Job drawing, mm, ordinate dimensions from the low corner. One solid piece. A direction names the side the tool comes from. Round coordinates to 2 decimals unless told otherwise and drop trailing zeros. Order: outer loops, then holes, each group sorted by start corner. A loop starts at its lowest first (then second) coordinate and runs counter-clockwise, first axis right, second up. Notation, with made-up numbers: (74, -30) -> (95, -30) arc R18 cw to (95, 2) -> close; hole circle Ø4 at (-23, 3.5). An arc over 180 degrees is marked (long way). Return JSON: item names as keys, results as strings. Group by question number.
Q1. Which spindle directions (+Z, -Z, +X, -X, +Y, -Y) get a long thin tool onto all of the face, cutting with end or side? Do the marked faces 4, 5 and 6. Say none if no direction does.
Q2. Mould opens along Y. For the marked faces 1, 2 and 3 say: +Y half, -Y half, draft (parallel to the pull), parting line (faces both ways), or undercut.
Q3. Flat gauge pins, fed straight in: pin 1 (7.5 mm diameter, centred on x = 60, y = 17.5, fed in from +Z); pin 2 (5 mm diameter, centred on y = 8, z = 6, fed in from +X); pin 3 (1.5 mm diameter, centred on y = 21, z = 9, fed in from -X). Where does each tip first touch, or does it go through?
Q4. Cut at B-B (z = 33.5). Write the cut outline in (x, y).
Q5. Cut at D-D (y = 23). Write the cut outline in (x, z), then the cut area to 3 significant figures.
Q6. Cut at A-A (y = 14). Write the cut outline in (x, z).
Q7. Probe line 1 along Z through (x, y) = (44.25, 12.7) (3 decimals); line 2 along X through (y, z) = (8.75, 8); line 3 along X through (y, z) = (19, 21.5). List the from-to ranges inside material, lowest first.
Q8. Cut at C-C (x = 14). Write the cut outline in (y, z), then the cut area to 3 significant figures.
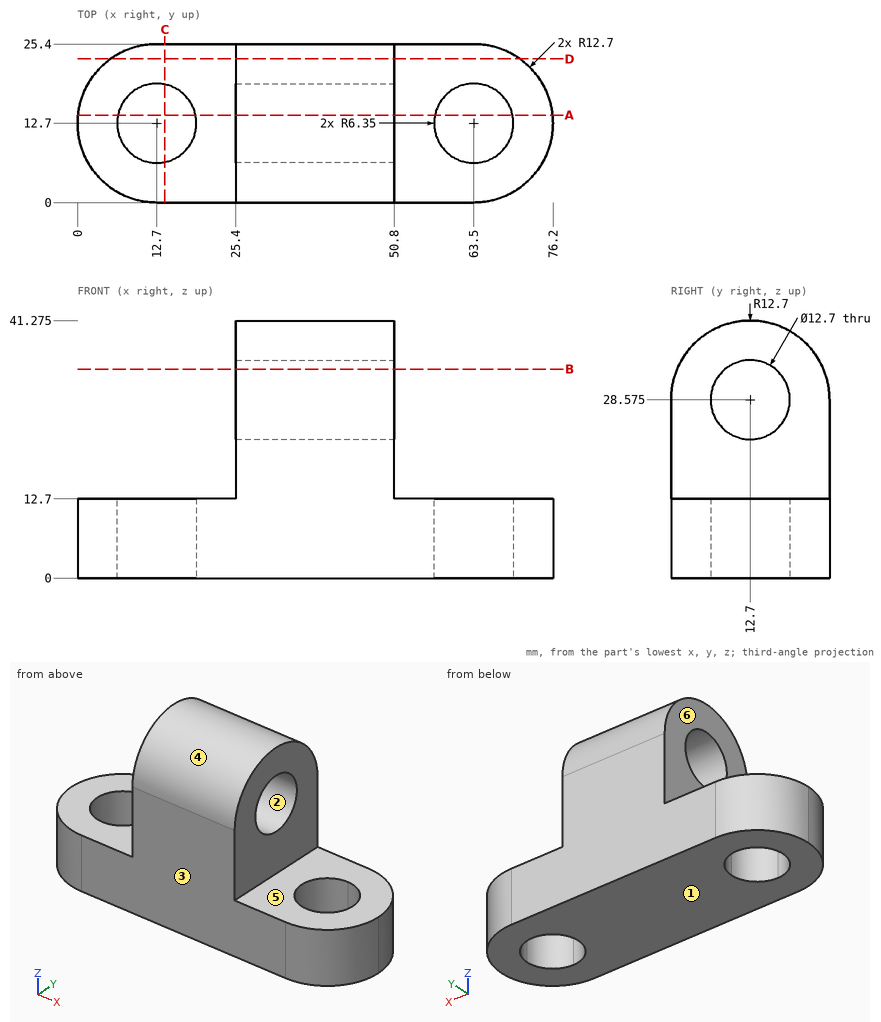
Solution:
{
 "1": {"face 4": "+Z, +X, -X", "face 5": "+Z, +X, +Y, -Y", "face 6": "+Z, -X, +Y, -Y"},
 "2": {"face 1": "draft", "face 2": "undercut", "face 3": "-Y half"},
 "3": {"pin 1": "stops at z = 12.7", "pin 2": "stops at x = 76.01", "pin 3": "stops at x = 2.49"},
 "4": {"outline": "(25.4, 0.99) -> (50.8, 0.99) -> (50.8, 8.69) -> (25.4, 8.69) -> close; (25.4, 16.71) -> (50.8, 16.71) -> (50.8, 24.41) -> (25.4, 24.41) -> close"},
 "5": {"outline": "(5.27, 0) -> (70.93, 0) -> (70.93, 12.7) -> (50.8, 12.7) -> (50.8, 36) -> (25.4, 36) -> (25.4, 12.7) -> (5.27, 12.7) -> close", "area": "1,430 mm²"},
 "6": {"outline": "(0.07, 0) -> (6.48, 0) -> (6.48, 12.7) -> (0.07, 12.7) -> close; (18.92, 0) -> (57.28, 0) -> (57.28, 12.7) -> (50.8, 12.7) -> (50.8, 22.36) -> (25.4, 22.36) -> (25.4, 12.7) -> (18.92, 12.7) -> close; (25.4, 34.79) -> (50.8, 34.79) -> (50.8, 41.21) -> (25.4, 41.21) -> close; (69.72, 0) -> (76.13, 0) -> (76.13, 12.7) -> (69.72, 12.7) -> close"},
 "7": {"line 1": "z = 0 to 22.225, 34.925 to 41.275", "line 2": "x = 0.63 to 7.73, 17.67 to 58.53, 68.47 to 75.57", "line 3": "x = 25.4 to 50.8"},
 "8": {"outline": "(0, 0) -> (6.48, 0) -> (6.48, 12.7) -> (0, 12.7) -> close; (18.92, 0) -> (25.4, 0) -> (25.4, 12.7) -> (18.92, 12.7) -> close", "area": "165 mm²"}
}
